Geometry check sheet. Reference: the model listing, model coordinates, mm. A direction names the side the tool comes from. Coordinates: 2 decimals unless noted, no trailing zeros. Order: outer loops, then holes, each group sorted by start corner. A loop starts at its lowest first (then second) coordinate and runs counter-clockwise, first axis right, second up. Notation, with made-up numbers: (36, 69.25) - (61, 69.25) arc R6 cw to (61, 77.25) - close; hole circle Ø9 at (-26, -29). An arc over 180 degrees is marked (long way). Use CSV: the item, a comma, the result in double quotes. Start each with the question number.
1) Tool access check on faces 1 (the flat face through (-1, -12.7, 0)), 2 (the flat face through (47.625, -1, 0)). Record the directions out of +Z, -Z, +X, -X, +Y, -Y that give a thin tool (end or side, any length) a straight path to the whole face; none if there is none.
2) Sectioned sample at A-A, the plane z = 0. Record the cut outline in (x, y) (3 decimals), and give its area (3 significant figures).
3) Draft check along X on faces 3 (the flat face through (-49, 12.7, 0)), 4 (the conical face through (31.892, -12.322, -0.737)), 5 (the flat face through (-50.8, 0, 0)). Enter one of: released by +X, released by -X, zero draft, split by the parting line, or undercut.
4) Sectioned sample at B-B, the plane y = 8.5. Record the cut outline in (x, z) (3 decimals).
5) Thickness scan on probe 1 along X at (y, z) = (-12.65, 0); probe 2 along X at (y, z) = (8.25, -9) (3 decimals); probe 3 along Y at (x, z) = (50.1, 0). Record the ranges inside material, lowest first. Write a range as [from, to].
6) Depth check by flat-ended pin: P1, Ø2, axis at x = 34.5, z = -7.5, coming from the +Y side (3 decimals); P2, Ø8.5, axis at x = -28.575, z = 0, coming from the +Y side. Enter the tip coordinate at first touch or a pass-through.
7) Sectioned sample at C-C, the plane z = 22. Record the cut outline in (x, y) (3 decimals).
8) Sectioned sample at D-D, the plane x = 11.5. Record the cut outline in (y, z) (3 decimals).
from build123d import *

# Parameters (mm, degrees)
BOSS_EXTRUDE2_DEPTH                  = 25.4
F_1_4_0_25_DIAMETER_HOLE1_AT_2_COUNT = 2
F_1_4_0_25_DIAMETER_HOLE1_AT_2_PITCH = 57.15
F_5_32_0_15625_DIAMETER_HOLE1_D      = 3.96875


with BuildPart() as part:
    # Sketch3 → Boss-Extrude2 (new, symmetric)
    with BuildSketch(Plane.XY):
        Polygon((-50.8, 12.7), (-50.8, -12.7), (50.8, -12.7), (50.8, 12.7), (47.625, 12.7), (47.625, -9.525), (-47.625, -9.525), (-47.625, 12.7), align=None)
    extrude(amount=BOSS_EXTRUDE2_DEPTH, both=True)

    # Sketch6 → 1/4 (0.25) Diameter Hole1 (revolve, cut)
    with BuildSketch(Plane(origin=(-28.575, -9.525, 0), x_dir=(0, 0, 1), z_dir=(1, 0, 0))):
        Polygon((0, 0), (0, 3.175), (3.175, 3.175), (3.175, 2.983838288), (6.731, 0), align=None)
    f_1_4_0_25_diameter_hole1 = revolve(axis=Axis((-28.575, -3.175, 0), (0, -1, 0)), mode=Mode.SUBTRACT)

    # 1/4 (0.25) Diameter Hole1 at 2: 1/4 (0.25) Diameter Hole1 ×2
    with Locations(*[(i * F_1_4_0_25_DIAMETER_HOLE1_AT_2_PITCH, 0, 0) for i in range(1, F_1_4_0_25_DIAMETER_HOLE1_AT_2_COUNT)]):
        add(f_1_4_0_25_diameter_hole1, mode=Mode.SUBTRACT)

    # 5/32 (0.15625) Diameter Hole1 (through all)
    with Locations(Plane(origin=(50.8, 0, 0), x_dir=(0, 0, -1), z_dir=(1, 0, 0))):
        with Locations((0, 3.215843377)):
            Hole(F_5_32_0_15625_DIAMETER_HOLE1_D / 2)


solid = part.part
Evaluation:
1,face 1,"+Z, -Z, +X, -X, -Y"
1,face 2,"+Z, -Z, +Y"
2,outline,"(-50.8, -12.7) - (-31.75, -12.7) - (-31.75, -12.509) - (-35.306, -9.525) - (-47.625, -9.525) - (-47.625, 1.231) - (-50.8, 1.231) - close; (-50.8, 5.2) - (-47.625, 5.2) - (-47.625, 12.7) - (-50.8, 12.7) - close; (-25.4, -12.7) - (25.4, -12.7) - (25.4, -12.509) - (21.844, -9.525) - (-21.844, -9.525) - (-25.4, -12.509) - close; (31.75, -12.7) - (50.8, -12.7) - (50.8, 1.231) - (47.625, 1.231) - (47.625, -9.525) - (35.306, -9.525) - (31.75, -12.509) - close; (47.625, 5.2) - (50.8, 5.2) - (50.8, 12.7) - (47.625, 12.7) - close"
2,area,"377 mm²"
3,face 3,"zero draft"
3,face 4,"undercut"
3,face 5,"released by -X"
4,outline,"(-50.8, -25.4) - (-47.625, -25.4) - (-47.625, 25.4) - (-50.8, 25.4) - close; (47.625, -25.4) - (50.8, -25.4) - (50.8, 25.4) - (47.625, 25.4) - close"
5,probe 1,"[-50.8, -31.75], [-25.4, 25.4], [31.75, 50.8]"
5,probe 2,"[-50.8, -47.625], [47.625, 50.8]"
5,probe 3,"[-12.7, 1.23], [5.2, 12.7]"
6,P1,"y = -9.525"
6,P2,"y = -11.61"
7,outline,"(-50.8, -12.7) - (50.8, -12.7) - (50.8, 12.7) - (47.625, 12.7) - (47.625, -9.525) - (-47.625, -9.525) - (-47.625, 12.7) - (-50.8, 12.7) - close"
8,outline,"(-12.7, -25.4) - (-9.525, -25.4) - (-9.525, 25.4) - (-12.7, 25.4) - close"
